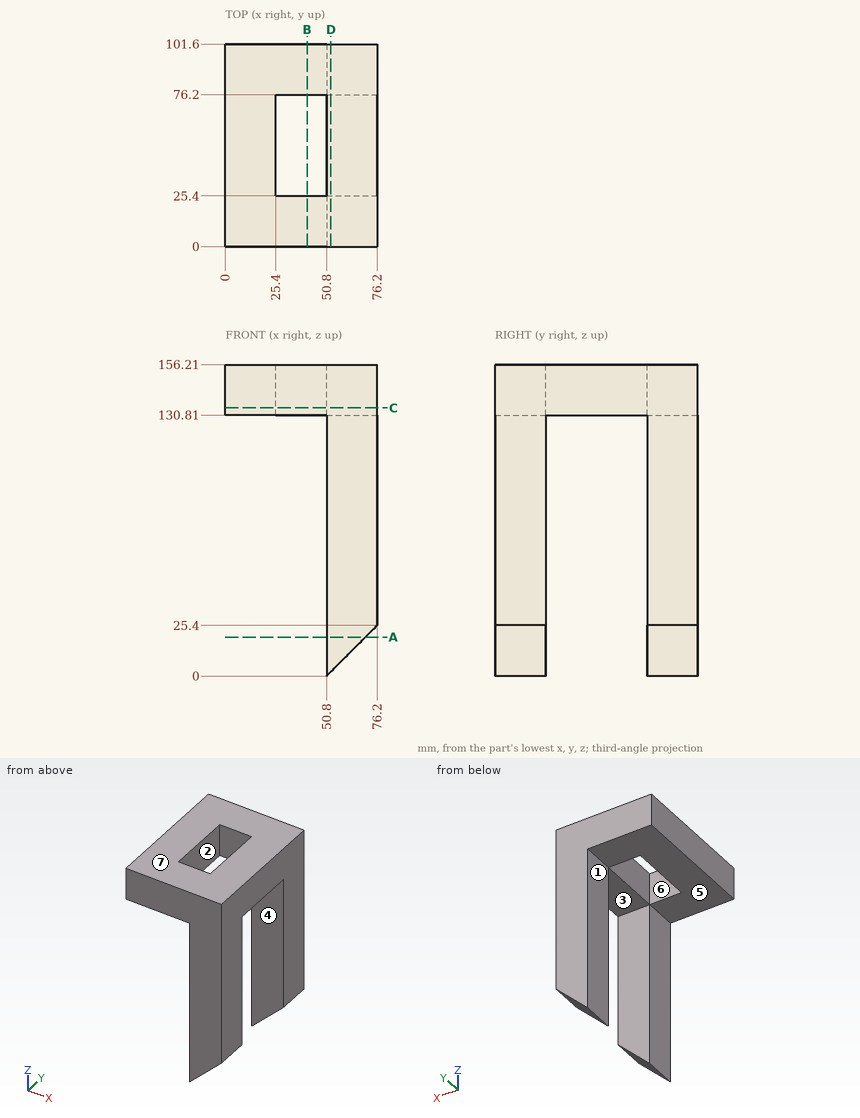
Source: three-view drawing plus pictorial views. Frame: mm from the lowest corner of the part. A direction names the side the tool comes from. Round coordinates to 2 decimals unless told otherwise and drop trailing zeros. Loops run counter-clockwise (first coordinate to the right, second up) from the corner with the lowest first, then second, coordinate; pieces in that order, holes last.
Item 1: Mould query, pull axis X, two halves, no side actions, for the marked faces 1, 2 and 3. Classes: released by +X, released by -X, zero draft, split by the parting line, or undercut.
Checked values:
face 1: released by -X
face 2: undercut
face 3: zero draft
Item 2: Reachability of the marked faces 4, 5, 6 and 7 from +Z, -Z, +X, -X, +Y, -Y: full face, straight path, thin tool, end or side. Return the list, or none.
Checked values:
face 4: -Z, +X, -X
face 5: -Z, -X, +Y, -Y
face 6: +Z, -Z
face 7: +Z, +X, -X, +Y, -Y
Item 3: Section D-D, the plane x = 53. Output: boundary loops of the cut face in (y, z), plus the area to 3 significant figures.
Checked values:
outline: (0, 2.2) - (25.4, 2.2) - (25.4, 130.81) - (76.2, 130.81) - (76.2, 2.2) - (101.6, 2.2) - (101.6, 156.21) - (0, 156.21) - close
area: 9,110 mm2
Item 4: Section A-A, the plane z = 19.5. Output: boundary loops of the cut face in (x, y).
Checked values:
outline: (50.8, 0) - (70.3, 0) - (70.3, 25.4) - (50.8, 25.4) - close; (50.8, 76.2) - (70.3, 76.2) - (70.3, 101.6) - (50.8, 101.6) - close
Item 5: Line query: L1, parallel to Y at x = 58.5, z = 99; L2, parallel to X at y = 19, z = 51.5; L3, parallel to Z at x = 25.5, y = 11. Output: solid intervals per line, ascending.
Checked values:
L1: y = 0 to 25.4, 76.2 to 101.6
L2: x = 50.8 to 76.2
L3: z = 130.81 to 156.21
Item 6: Section C-C, the plane z = 134.5. Output: boundary loops of the cut face in (x, y).
Checked values:
outline: (0, 0) - (76.2, 0) - (76.2, 101.6) - (0, 101.6) - close; hole (25.4, 25.4) - (50.8, 25.4) - (50.8, 76.2) - (25.4, 76.2) - close
Item 7: Section B-B, the plane x = 41. Output: boundary loops of the cut face in (y, z).
Checked values:
outline: (0, 130.81) - (25.4, 130.81) - (25.4, 156.21) - (0, 156.21) - close; (76.2, 130.81) - (101.6, 130.81) - (101.6, 156.21) - (76.2, 156.21) - close
Item 8: Contact query for flat-ended pins moving along their axis: P1, Ø20.5, axis at y = 9, z = 36, coming from the -X side; P2, Ø6, axis at y = 25.5, z = 96.5, coming from the +X side; P3, Ø20.5, axis at x = 60.5, y = 41.5, coming from the -Z side; P4, Ø5, axis at x = 47, y = 66, coming from the +Z side. Output: stop coordinate, or through.
Checked values:
P1: stops at x = 50.8
P2: stops at x = 76.2
P3: stops at z = 130.81
P4: passes through
